```python
from build123d import *

# Parameters (mm, degrees)
F0_W           = 150
F0_H           = 200
F0_W_2         = 137.5
F0_H_2         = 187.5
F1_DEPTH       = 10
F0_R           = 5
F2_DEPTH       = 5
F0_R_2         = 2.5
F3_DEPTH       = 2
F5_D           = 3
F5_CSINK_D     = 5
F5_CSINK_ANGLE = 90


with BuildPart() as f1:
    # F0 (on Top) → F1 (new body)
    with BuildSketch(Plane.XY):
        with Locations((-0.025054, 0.008351)):
            Rectangle(F0_W, F0_H)
        with Locations((-0.025054, 0.008351)):
            Rectangle(F0_W_2, F0_H_2, mode=Mode.SUBTRACT)
    extrude(amount=F1_DEPTH)

    # F0 (on Top) → F2 (join)
    with BuildSketch(Plane.XY):
        with Locations((-0.025054, 0.008351)):
            Rectangle(F0_W_2, F0_H_2)
        Polygon((-62.525054, 62.508351), (-62.525054, 87.508351), (-37.525054, 87.508351), (37.474946, 87.508351), (62.474946, 87.508351), (62.474946, 62.508351), (62.474946, -62.491649), (62.474946, -87.491649), (37.474946, -87.491649), (-37.525054, -87.491649), (-62.525054, -87.491649), (-62.525054, -62.491649), align=None, mode=Mode.SUBTRACT)
        Polygon((-37.525054, 87.508351), (-62.525054, 87.508351), (-62.525054, 62.508351), align=None)
        with Locations((-56.275054, 81.258351)):
            Circle(F0_R, mode=Mode.SUBTRACT)
        Polygon((62.474946, 87.508351), (37.474946, 87.508351), (62.474946, 62.508351), align=None)
        with Locations((56.224946, 81.258351)):
            Circle(F0_R, mode=Mode.SUBTRACT)
        Polygon((62.474946, -87.491649), (62.474946, -62.491649), (37.474946, -87.491649), align=None)
        with Locations((56.224946, -81.241649)):
            Circle(F0_R, mode=Mode.SUBTRACT)
        Polygon((-37.525054, -87.491649), (-62.525054, -62.491649), (-62.525054, -87.491649), align=None)
        with Locations((-56.275054, -81.241649)):
            Circle(F0_R, mode=Mode.SUBTRACT)
    extrude(amount=F2_DEPTH)

    # F0 (on Top) → F3 (join)
    with BuildSketch(Plane.XY):
        with Locations((-56.275054, 81.258351)):
            Circle(F0_R)
        with Locations((-56.275054, 81.258351)):
            Circle(F0_R_2, mode=Mode.SUBTRACT)
        with Locations((56.224946, 81.258351)):
            Circle(F0_R)
        with Locations((56.224946, 81.258351)):
            Circle(F0_R_2, mode=Mode.SUBTRACT)
        with Locations((56.224946, -81.241649)):
            Circle(F0_R)
        with Locations((56.224946, -81.241649)):
            Circle(F0_R_2, mode=Mode.SUBTRACT)
        with Locations((-56.275054, -81.241649)):
            Circle(F0_R)
        with Locations((-56.275054, -81.241649)):
            Circle(F0_R_2, mode=Mode.SUBTRACT)
    extrude(amount=F3_DEPTH)

    # F5 (through all)
    with Locations(Plane.XY.offset(5)):
        with Locations((-62.525054, 87.508351), (62.474946, 87.508351), (62.474946, -87.491649), (-62.525054, -87.491649)):
            CounterSinkHole(F5_D / 2, F5_CSINK_D / 2, counter_sink_angle=F5_CSINK_ANGLE)


solid = f1.part
```
CAD build for the part. Positions are in the model's coordinates, mm. A direction names the side the tool comes from. Round coordinates to 2 decimals unless told otherwise and drop trailing zeros. Write each loop counter-clockwise with the first axis right and the second up, starting at its lowest first coordinate (ties: lowest second). Pieces come first, ordered by that corner, then holes. Notation, with made-up numbers: (15, -11) - (59, -11) arc R24 ccw to (59, -1) - close; hole circle Ø8 at (39.25, 10). An arc over 180 degrees is marked (long way). Return JSON: item names as keys, results as strings. Group by question number.
Item 1: Flat gauge pins, fed straight in: pin 1 Ø2.5 at (x, y) = (-62.53, 87.51) entering from -Z; pin 2 Ø6 at (x, y) = (-56.28, -81.24) entering from +Z; pin 3 Ø8 at (x, y) = (55, -83) entering from +Z. Where does each tip first touch, or does it go through?
Item 2: Band-saw the part on A-A on x = -23. List the corners of the cut face in (y, z), plus the area to 4 significant figures.
Item 3: 3-axis set-ups, long thin cutter, end or side, ignore diameter. For faces 4 (the face through (-51.656, -83.157, 3.479)), 5 (the face through (49.8, 75.183, 2.465)), 6 (the face through (74.975, -1, 5)): which of +Z, -Z, +X, -X, +Y, -Y reach the whole face in a straight line?
Item 4: Mould opens along Y. For faces 1 (the face through (-62.525, -1, 2)), 2 (the face through (-1, 100.008, 5)), 3 (the face through (66, 0, 0)) say: +Y half, -Y half, draft (parallel to the pull), parting line (faces both ways), or undercut.
Item 5: Probe probe 1 along X at (y, z) = (42, 2.5); probe 2 along Y at (x, z) = (-18.5, 2); probe 3 along X at (y, z) = (-68.5, 6.25). List the from-to ranges inside material, lowest first.
Item 6: Band-saw the part on B-B on y = 59. List the corners of the cut face in (x, z), plus the area to 4 significant figures.
Resolved:
{
 "1": {"pin 1": "passes through", "pin 2": "stops at z = 2", "pin 3": "stops at z = 5"},
 "2": {"outline": "(-99.99, 0) - (-87.49, 0) - (-87.49, 5) - (-93.74, 5) - (-93.74, 10) - (-99.99, 10) - close; (87.51, 0) - (100.01, 0) - (100.01, 10) - (93.76, 10) - (93.76, 5) - (87.51, 5) - close", "area": "187.5 mm²"},
 "3": {"face 4": "+Z", "face 5": "+Z, -Z", "face 6": "+Z, -Z, +X, +Y, -Y"},
 "4": {"face 1": "undercut", "face 2": "+Y half", "face 3": "draft"},
 "5": {"probe 1": "x = -75.03 to -62.53, 62.47 to 74.97", "probe 2": "y = -99.99 to -87.49, 87.51 to 100.01", "probe 3": "x = -75.03 to -68.78, 68.72 to 74.97"},
 "6": {"outline": "(-75.03, 0) - (-62.53, 0) - (-62.53, 5) - (-68.78, 5) - (-68.78, 10) - (-75.03, 10) - close; (62.47, 0) - (74.97, 0) - (74.97, 10) - (68.72, 10) - (68.72, 5) - (62.47, 5) - close", "area": "187.5 mm²"}
}
